```python
from build123d import *

# Parameters (mm, degrees)
SKETCH1_W           = 80
SKETCH1_H           = 60
BOSS_EXTRUDE1_DEPTH = 5
SKETCH2_W           = 5
SKETCH2_H           = 60
BOSS_EXTRUDE2_DEPTH = 25
SKETCH3_R           = 1.8
CUT_EXTRUDE1_DEPTH  = 30
CUT_EXTRUDE2_DEPTH  = 30
FILLET1_R           = 5
SKETCH6_R           = 2.5
CUT_EXTRUDE3_DEPTH  = 30
SKETCH8_W           = 5
SKETCH8_H           = 20
SKETCH8_H_2         = 4
BOSS_EXTRUDE3_DEPTH = 4
FILLET3_R           = 1.5
BOSS_EXTRUDE4_DEPTH = 3
FILLET4_R           = 5
FILLET5_R           = 2


with BuildPart() as part:
    # Sketch1 → Boss-Extrude1 (new body)
    with BuildSketch(Plane(origin=(0, 0, 0), x_dir=(1, 0, 0), z_dir=(0, 1, 0))):
        Rectangle(SKETCH1_W, SKETCH1_H)
    extrude(amount=BOSS_EXTRUDE1_DEPTH)

    # Sketch2 → Boss-Extrude2 (add)
    with BuildSketch(Plane(origin=(0, 5, 0), x_dir=(1, 0, 0), z_dir=(0, 1, 0))):
        with Locations((17.5, 0)):
            Rectangle(SKETCH2_W, SKETCH2_H)
    extrude(amount=BOSS_EXTRUDE2_DEPTH)

    # Sketch3 → Cut-Extrude1 (cut)
    with BuildSketch(Plane.ZY.offset(-15)):
        with Locations((-22.5, 18)):
            Circle(SKETCH3_R)
        with Locations((22.5, 18)):
            Circle(SKETCH3_R)
    extrude(amount=-CUT_EXTRUDE1_DEPTH, mode=Mode.SUBTRACT)

    # Sketch5 → Cut-Extrude2 (cut)
    with BuildSketch(Plane(origin=(0, 5, 0), x_dir=(1, 0, 0), z_dir=(0, 1, 0))):
        with BuildLine():
            Line((40, 30), (36.243947384, 30))
            ThreePointArc((36.243947384, 30), (39.057335538, 15.117108944), (40, 0))
            Line((40, 0), (40, 30))
        make_face()
        with BuildLine():
            Line((40, -30), (40, 0))
            ThreePointArc((40, 0), (39.057335538, -15.117108944), (36.243947384, -30))
            Line((36.243947384, -30), (40, -30))
        make_face()
    extrude(amount=-CUT_EXTRUDE2_DEPTH, mode=Mode.SUBTRACT)

    # Fillet1
    fillet1_edges = [part.edges().sort_by_distance(p)[0] for p in [
        (17.5, 30, 30),
        (17.5, 30, -30),
        (36.243947384, 2.5, 30),
        (36.243947384, 2.5, -30),
        (-40, 2.5, -30),
        (-40, 2.5, 30),
    ]]
    fillet(fillet1_edges, radius=FILLET1_R)

    # Sketch6 → Cut-Extrude3 (cut)
    with BuildSketch(Plane(origin=(0, 5, 0), x_dir=(1, 0, 0), z_dir=(0, 1, 0))):
        with Locations(Location((-30, 20, 0), (0, 0, 270))):
            Circle(SKETCH6_R)
        with Locations(Location((-30, -20, 0), (0, 0, 270))):
            Circle(SKETCH6_R)
        with Locations(Location((-10, 20, 0), (0, 0, 270))):
            Circle(SKETCH6_R)
        with Locations(Location((-10, -20, 0), (0, 0, 270))):
            Circle(SKETCH6_R)
    extrude(amount=-CUT_EXTRUDE3_DEPTH, mode=Mode.SUBTRACT)

    # Sketch8 → Boss-Extrude3 (add)
    with BuildSketch(Plane(origin=(0, 5, 0), x_dir=(1, 0, 0), z_dir=(0, 1, 0))):
        with Locations((-30, 0)):
            Rectangle(SKETCH8_W, SKETCH8_H)
        with Locations((-30, 28)):
            Rectangle(SKETCH8_W, SKETCH8_H_2)
        with Locations((-30, -28)):
            Rectangle(SKETCH8_W, SKETCH8_H_2)
    extrude(amount=BOSS_EXTRUDE3_DEPTH)

    # Fillet3
    fillet3_edges = [part.edges().sort_by_distance(p)[0] for p in [
        (-32.5, 9, 0),
        (-27.5, 9, 0),
        (-27.5, 9, -28),
        (-32.5, 9, -28),
        (-27.5, 9, 28),
        (-32.5, 9, 28),
    ]]
    fillet(fillet3_edges, radius=FILLET3_R)

    # Sketch9 → Boss-Extrude4 (add)
    with BuildSketch(Plane.XY.offset(30)):
        Polygon((15, 25), (5, 5), (15, 5), align=None)
    boss_extrude4 = extrude(amount=-BOSS_EXTRUDE4_DEPTH)

    # Mirror1: Boss-Extrude4 across plane
    add(boss_extrude4.mirror(Plane.XY))

    # Fillet4
    fillet4_edges = [part.edges().sort_by_distance(p)[0] for p in [
        (15, 5, 0),
    ]]
    fillet(fillet4_edges, radius=FILLET4_R)

    # Fillet5
    fillet5_edges = [part.edges().sort_by_distance(p)[0] for p in [
        (20, 5, 0),
    ]]
    fillet(fillet5_edges, radius=FILLET5_R)


solid = part.part
```
Can you work these out from the model? Positions are in its coordinate system, mm. A direction names the side the tool comes from. Give positions to 0.01 mm unless a question says otherwise; leave off trailing zeros. Loops run counter-clockwise (first coordinate to the right, second up) from the corner with the lowest first, then second, coordinate; pieces in that order, holes last. Notation, with made-up numbers: M 55,48 L 70,48 A21 ccw 70,86 Z; hole C 32.5,-30.5 d9. An arc over 180 degrees is marked long. Answer in a Markdown table with one row per item.
1. Suppose I cut it at D-D on x = -10. Write out the boundary of the cut face in (y, z), plus the area to 3 significant figures.
Taken from the geometry:
| item | result |
|---|---|
| outline | M 0,-30 L 5,-30 L 5,-22.5 L 0,-22.5 Z; M 0,-17.5 L 5,-17.5 L 5,17.5 L 0,17.5 Z; M 0,22.5 L 5,22.5 L 5,30 L 0,30 Z |
| area | 250 mm² |
2. Thinking about a two-plate mould opening in Y: for faces 1 (the flat face through (10, 15, 29)), 2 (the flat face through (-27.5, 6, 28)), 3 (the cylindrical face through (17.465, 19.785, -22.734)), which applies, released by +Y, released by -Y, zero draft, split by the parting line, or undercut?
Taken from the geometry:
| item | result |
|---|---|
| face 1 | released by +Y |
| face 2 | zero draft |
| face 3 | undercut |
3. Suppose I cut it at C-C on z = -7. Write out the boundary of the cut face in (x, y), plus the area to 3 significant figures.
Taken from the geometry:
| item | result |
|---|---|
| outline | M -40,0 L 39.8,0 L 39.8,5 L 22,5 A2 cw 20,7 L 20,30 L 15,30 L 15,10 A5 cw 10,5 L -27.5,5 L -27.5,7.5 A1.5 ccw -29,9 L -31,9 A1.5 ccw -32.5,7.5 L -32.5,5 L -40,5 Z |
| area | 549 mm² |
4. For pin 1 Ø1 at (y, z) = (18.5, -10.5) entering from +X; pin 2 Ø1.2 at (y, z) = (6.5, 27.5) entering from +X; pin 3 Ø3 at (y, z) = (21.5, -5.5) entering from -X; pin 4 Ø20 at (x, z) = (29, 6.5) entering from +Y, each with a flat end and sliding along its axis, tell me the tip position at first contact or that it passes through.
Taken from the geometry:
| item | result |
|---|---|
| pin 1 | stops at x = 20 |
| pin 2 | stops at x = 20.33 |
| pin 3 | stops at x = 15 |
| pin 4 | stops at y = 30 |
5. Suppose I cut it at B-B on y = 3.25. Write out the boundary of the cut face in (x, z).
Taken from the geometry:
| item | result |
|---|---|
| outline | M -40,-25 A5 ccw -35,-30 L 32.29,-30 A5 ccw 37.17,-26.07 A121.68 ccw 37.17,26.07 A5 ccw 32.29,30 L -35,30 A5 ccw -40,25 Z; hole C -30,-20 d5; hole C -30,20 d5; hole C -10,-20 d5; hole C -10,20 d5 |
6. If I drill on line 1 along Z through (x, y) = (10, 10); line 2 along X through (y, z) = (1.55, -20); line 3 along Y through (x, z) = (36, -8), over which ranges is the centre line in solid material (lowest first)?
Taken from the geometry:
| item | result |
|---|---|
| line 1 | z = -30 to -27, 27 to 30 |
| line 2 | x = -40 to -32.5, -27.5 to -12.5, -7.5 to 38.35 |
| line 3 | y = 0 to 5 |
7. Suppose I cut it at A-A on x = -30. Write out the boundary of the cut face in (y, z), plus the area to 3 significant figures.
Taken from the geometry:
| item | result |
|---|---|
| outline | M 0,-30 L 9,-30 L 9,-26 L 5,-26 L 5,-22.5 L 0,-22.5 Z; M 0,-17.5 L 5,-17.5 L 5,-10 L 9,-10 L 9,10 L 5,10 L 5,17.5 L 0,17.5 Z; M 0,22.5 L 5,22.5 L 5,26 L 9,26 L 9,30 L 0,30 Z |
| area | 362 mm² |
8. Which directions (+Z, -Z, +X, -X, +Y, -Y) give clear straight access to the entire face, cutting with the end or side of a thin tool? Please do faces 4 (the flat face through (-32.5, 6, 28)), 5 (the flat face through (12, 11, 27)), 6 (the flat face through (31, 5, 0)).
Taken from the geometry:
| item | result |
|---|---|
| face 4 | +Z, -Z, -X, +Y |
| face 5 | +Y |
| face 6 | +Z, -Z, +X, +Y |
